Model file for the job. Use its own axes, mm. A direction names the side the tool comes from. Coordinates: 2 decimals unless noted, no trailing zeros. Write each loop counter-clockwise with the first axis right and the second up, starting at its lowest first coordinate (ties: lowest second). Pieces come first, ordered by that corner, then holes. Notation, with made-up numbers: M 11,24 L 69,24 A22 cw 69,31 Z; hole C 5.5,33.5 d10. An arc over 180 degrees is marked long. Answer in a Markdown table with one row per item. Add a question column.
```python
from build123d import *

# Parameters (mm, degrees)
F0_R     = 4.7625
F1_DEPTH = 7.9502
F2_R     = 5.3975
F2_R_2   = 4.7625
F3_DEPTH = 1.27
F4_R     = 3.175
F5_DEPTH = 12.7


with BuildPart() as f1:
    # F0 (on Top) → F1 (new body)
    with BuildSketch(Plane.XY):
        Circle(F0_R)
    extrude(amount=F1_DEPTH)

    # F2 (on face) → F3 (join)
    with BuildSketch(Plane.XY.offset(7.9502)):
        Circle(F2_R)
        Circle(F2_R_2, mode=Mode.SUBTRACT)
    extrude(amount=-F3_DEPTH)

    # F4 (on face) → F5 (join)
    with BuildSketch(Plane.XY.offset(7.9502)):
        Circle(F4_R)
    extrude(amount=F5_DEPTH)


solid = f1.part
```
1) Drill centre lines: probe 1 along Z at (x, y) = (-3, 4); probe 2 along Z at (x, y) = (-3.5, -1.5); probe 3 along X at (y, z) = (-3.75, 3). Where is each one in solid material? Low to high.
2) Slice it at C-C (z = 8.25). Give the cut face in (x, y) (3 decimals), then the cut area to 3 significant figures.
3) Slice it at A-A (y = 0). Give the cut face in (x, z) (1 decimal), then the cut area to 3 significant figures.
4) Which spindle directions (+Z, -Z, +X, -X, +Y, -Y) get a long thin tool onto all of the face, cutting with end or side? Do faces 1 (the face through (-0.69, -3.1, 14.21)), 2 (the face through (0, 0, 20.65)), 3 (the face through (0, -5, 6.68)). Say none if no direction does.
5) Slice it at D-D (x = -4.25). Give the cut face in (y, z).
6) Flat gauge pins, fed straight in: pin 1 Ø4 at (x, z) = (2.5, 3) entering from -Y; pin 2 Ø1.5 at (y, z) = (4, 13.5) entering from -X; pin 3 Ø4 at (y, z) = (3, 5.5) entering from -X; pin 4 Ø5 at (y, z) = (2.5, 9) entering from -X. Where does each tip first touch, or does it go through?
Ans:
| question | item | result |
|---|---|---|
| 1 | probe 1 | z = 6.68 to 7.95 |
| 1 | probe 2 | z = 0 to 7.95 |
| 1 | probe 3 | x = -2.94 to 2.94 |
| 2 | outline | C 0,0 d6.35 |
| 2 | area | 31.7 mm2 |
| 3 | outline | M -5.4,6.7 L -4.8,6.7 L -4.8,0 L 4.8,0 L 4.8,6.7 L 5.4,6.7 L 5.4,8 L 3.2,8 L 3.2,20.7 L -3.2,20.7 L -3.2,8 L -5.4,8 Z |
| 3 | area | 158 mm2 |
| 4 | face 1 | +Z |
| 4 | face 2 | +Z, +X, -X, +Y, -Y |
| 4 | face 3 | -Z |
| 5 | outline | M -3.33,6.68 L -2.15,6.68 L -2.15,0 L 2.15,0 L 2.15,6.68 L 3.33,6.68 L 3.33,7.95 L -3.33,7.95 Z |
| 6 | pin 1 | stops at y = -4.74 |
| 6 | pin 2 | passes through |
| 6 | pin 3 | stops at x = -5.22 |
| 6 | pin 4 | stops at x = -5.39 |
